Part print with two shaded views. Sizes in mm from the minimum x, y, z corner. Coordinates: 2 decimals unless noted, no trailing zeros. Order: outer loops, then holes, each group sorted by start corner. A loop starts at its lowest first (then second) coordinate and runs counter-clockwise, first axis right, second up. Notation, with made-up numbers: M 38,-36 L 71,-36 A10 ccw 71,-31 Z; hole C 12,9.25 d11. An arc over 180 degrees is marked long. Answer in a Markdown table with one row per item. Add a question column.
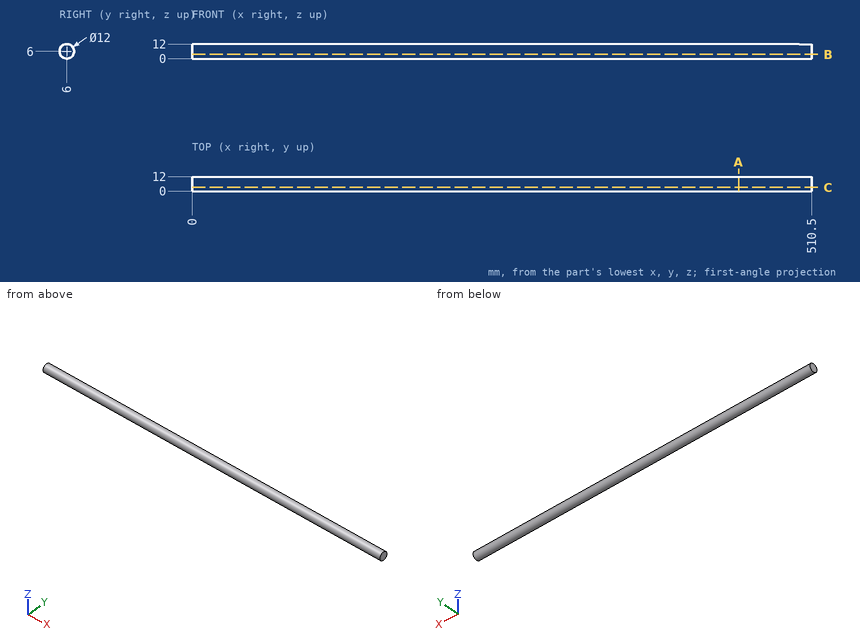
(1) Slice it at B-B (z = 3.5). List the corners of the cut face in (x, y), and give its area (3 significant figures).
(2) Drop a flat-ended pin along its axis: P1, Ø1.5, axis at x = 407, z = 7.5, coming from the +Y side. Give the stop position or say it passes through.
(3) Slice it at A-A (x = 450.5). List the corners of the cut face in (y, z).
(4) Slice it at C-C (y = 3). List the corners of the cut face in (x, z).
(5) Wall check: line 1 (Y direction, x = 381, z = 5.25); line 2 (Y direction, x = 113.5, z = 7); line 3 (Z direction, x = 155, y = 0.5). Give the ranges that are in metal, low to high.
Computed:
| question | item | result |
|---|---|---|
| 1 | outline | M 0,0.55 L 510.5,0.55 L 510.5,11.45 L 0,11.45 Z |
| 1 | area | 5,570 mm^2 |
| 2 | P1 | stops at y = 11.95 |
| 3 | outline | C 6,6 d12 |
| 4 | outline | M 0,0.8 L 510.5,0.8 L 510.5,11.2 L 0,11.2 Z |
| 5 | line 1 | y = 0.05 to 11.95 |
| 5 | line 2 | y = 0.08 to 11.92 |
| 5 | line 3 | z = 3.6 to 8.4 |
